```python
from build123d import *

# Parameters (mm, degrees)
SKETCH1_W       = 50.8
SKETCH1_H       = 12.7
EXTRUDE1_DEPTH  = 3.175
EXTRUDE2_DEPTH  = 4.175
SKETCH3_W       = 12.7
SKETCH3_H       = 3.175
EXTRUDE3_DEPTH  = 3.175
LPATTERN1_COUNT = 2
LPATTERN1_PITCH = 38.1


with BuildPart() as part:
    # Sketch1 → Extrude1 (new body)
    with BuildSketch(Plane.XY):
        with Locations((25.4, 6.35)):
            Rectangle(SKETCH1_W, SKETCH1_H)
    extrude(amount=EXTRUDE1_DEPTH)

    # Sketch2 → Extrude2 (cut, through all)
    with BuildSketch(Plane.XY.offset(3.175)):
        with BuildLine():
            Line((15.24, 9.2075), (35.56, 9.2075))
            ThreePointArc((35.56, 9.2075), (38.4175, 6.35), (35.56, 3.4925))
            Line((35.56, 3.4925), (15.24, 3.4925))
            ThreePointArc((15.24, 3.4925), (12.3825, 6.35), (15.24, 9.2075))
        make_face()
    extrude(amount=-EXTRUDE2_DEPTH, mode=Mode.SUBTRACT)

    # Sketch3 → Extrude3 (add)
    with BuildSketch(Plane(origin=(0, 12.7, 0), x_dir=(1, 0, 0), z_dir=(0, 1, 0))):
        with Locations((6.35, -1.5875)):
            Rectangle(SKETCH3_W, SKETCH3_H)
    extrude3 = extrude(amount=EXTRUDE3_DEPTH)

    # LPattern1: Extrude3 ×2
    with Locations(*[(i * LPATTERN1_PITCH, 0, 0) for i in range(1, LPATTERN1_COUNT)]):
        add(extrude3)


solid = part.part
```
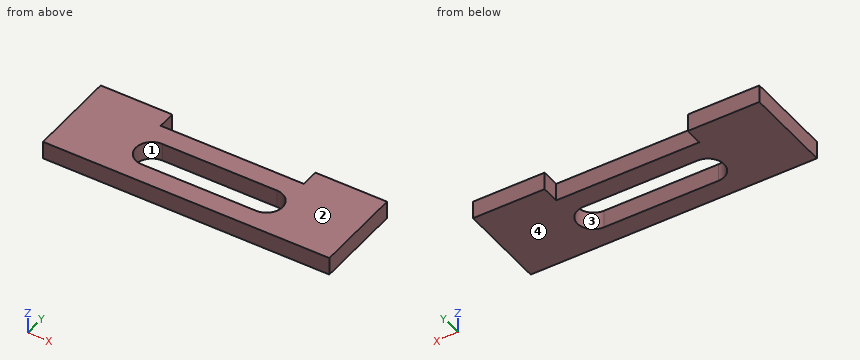
Source: CAD feature listing. Evaluate the final solid. Frame: model axes, mm. Face numbers are marked on the shaded views. A direction names the side the tool comes from. Give positions to 0.01 mm unless a question says otherwise; leave off trailing zeros. Order: outer loops, then holes, each group sorted by start corner. A loop starts at its lowest first (then second) coordinate and runs counter-clockwise, first axis right, second up.
(1) Section query B-B (x = 31). Return the cut outline in (y, z) (1 decimal).
(2) Pull-direction query (X, two-part tool) for the marked faces 3 and 4; classes: +X half, -X half, draft (parallel to the pull), parting line (faces both ways), or undercut.
(3) Material intervals for line 1 along Y through (x, z) = (35, 0.35); line 2 along X through (y, z) = (13, 1.1); line 3 along X through (y, z) = (6.5, 1.5), sorted ascending.
(4) Section query A-A (y = 6.35). Return the cut outline in (x, z) (1 decimal), plus the area to 3 significant figures.
(5) Contact query for a flat-ended pin moving along its axis: P1, Ø1, axis at x = 32.5, z = 0.5, coming from the +Y side. Output: stop coordinate, or through.
(6) Access query for the marked faces 1 and 2. Directions: +Z, -Z, +X, -X, +Y, -Y. A direction counts if a zero-diameter tool reaches every point of the face in a straight line with its end or side. Return the directions, or none.
Outcome:
1. outline: (0, 0) - (3.5, 0) - (3.5, 3.2) - (0, 3.2) - close; (9.2, 0) - (12.7, 0) - (12.7, 3.2) - (9.2, 3.2) - close
2. face 3: undercut
2. face 4: draft
3. line 1: y = 0 to 3.49, 9.21 to 12.7
3. line 2: x = 0 to 12.7, 38.1 to 50.8
3. line 3: x = 0 to 12.39, 38.41 to 50.8
4. outline: (0, 0) - (12.4, 0) - (12.4, 3.2) - (0, 3.2) - close; (38.4, 0) - (50.8, 0) - (50.8, 3.2) - (38.4, 3.2) - close
4. area: 78.6 mm2
5. P1: stops at y = 12.7
6. face 1: +Z, -Z
6. face 2: +Z, +X, -X, +Y, -Y
